```python
from build123d import *

# Parameters (mm, degrees)
SKETCH1_W           = 3
SKETCH1_H           = 30
BOSS_EXTRUDE1_DEPTH = 3


with BuildPart() as part:
    # Sketch1 → Boss-Extrude1 (new body)
    with BuildSketch(Plane.XY):
        Polygon((-90, 0), (-86.5, 0), (-86.5, 3), (-70, 3), (-70, 35), (-8, 35), (-8, 3), (-6.5, 3), (-6.5, 0), (17, 0), (17, 3), (0, 59), (-3, 59), (-90, 33), align=None)
        with Locations((-1.5, 31)):
            Rectangle(SKETCH1_W, SKETCH1_H, mode=Mode.SUBTRACT)
    extrude(amount=BOSS_EXTRUDE1_DEPTH)


solid = part.part
```
Work out the finished part from the listing and answer in its coordinate system (mm). A direction names the side the tool comes from. Coordinates: 2 decimals unless noted, no trailing zeros. Loops run counter-clockwise (first coordinate to the right, second up) from the corner with the lowest first, then second, coordinate; pieces in that order, holes last. Notation, with made-up numbers: (57, 25.25) - (101, 25.25) arc R26 cw to (101, 57.25) - close; hole circle Ø6 at (73.5, -30). An arc over 180 degrees is marked (long way). Use a Markdown table: item, result.
Item 1: For faces 4 (the flat face through (-78, 3, 1)), 5 (the flat face through (-3, 31, 1)), 6 (the flat face through (-88, 0, 1)), determine the directions among +Z, -Z, +X, -X, +Y, -Y from which every point of the face is accessible in a straight line to the end or side of a thin tool.
Evaluation:
| item | result |
|---|---|
| face 4 | +Z, -Z, -Y |
| face 5 | +Z, -Z |
| face 6 | +Z, -Z, +X, -X, -Y |
Item 2: Find section D-D, the plane y = 5.5. Determine the outline of the cut face in (x, z), and give its area (3 significant figures).
Evaluation:
| item | result |
|---|---|
| outline | (-90, 0) - (-70, 0) - (-70, 3) - (-90, 3) - close; (-8, 0) - (16.24, 0) - (16.24, 3) - (-8, 3) - close |
| area | 133 mm2 |
Item 3: The mould has two halves that part along X. Classify faces 1 (the flat face through (-1, 59, 1)), 2 (the flat face through (-86.5, 1, 1)), 3 (the flat face through (17, 1, 1)): +X half, -X half, draft (parallel to the pull), parting line (faces both ways), or undercut.
Evaluation:
| item | result |
|---|---|
| face 1 | draft |
| face 2 | undercut |
| face 3 | +X half |
Item 4: Find section B-B, the plane y = 25. Determine the outline of the cut face in (x, z), and give its area (3 significant figures).
Evaluation:
| item | result |
|---|---|
| outline | (-90, 0) - (-70, 0) - (-70, 3) - (-90, 3) - close; (-8, 0) - (-3, 0) - (-3, 3) - (-8, 3) - close; (0, 0) - (10.32, 0) - (10.32, 3) - (0, 3) - close |
| area | 106 mm2 |
Item 5: Consider probe 1 along X at (y, z) = (28, 1.5); probe 2 along X at (y, z) = (27, 0.7); probe 3 along Y at (x, z) = (-82.5, 2.65). Determine where each line is inside the solid, lowest interval first. Write a range as from..to.
Evaluation:
| item | result |
|---|---|
| probe 1 | x = -90..-70, -8..-3, 0..9.41 |
| probe 2 | x = -90..-70, -8..-3, 0..9.71 |
| probe 3 | y = 3..35.24 |
Item 6: Given pin 1 Ø1.2 at (x, z) = (-7.5, 1) entering from -Y; pin 2 Ø0.9 at (y, z) = (27, 1) entering from +X; pin 3 Ø1.5 at (x, z) = (-68.5, 1.5) entering from -Y, each flat-ended and moving along its own axis, determine where each tip first touches the part or whether it passes through.
Evaluation:
| item | result |
|---|---|
| pin 1 | stops at y = 3 |
| pin 2 | stops at x = 9.85 |
| pin 3 | stops at y = 35 |
Item 7: Find section C-C, the plane y = 13. Determine the outline of the cut face in (x, z).
Evaluation:
| item | result |
|---|---|
| outline | (-90, 0) - (-70, 0) - (-70, 3) - (-90, 3) - close; (-8, 0) - (13.96, 0) - (13.96, 3) - (-8, 3) - close |
Item 8: Find section A-A, the plane z = 2.4. Determine the outline of the cut face in (x, y).
Evaluation:
| item | result |
|---|---|
| outline | (-90, 0) - (-86.5, 0) - (-86.5, 3) - (-70, 3) - (-70, 35) - (-8, 35) - (-8, 3) - (-6.5, 3) - (-6.5, 0) - (17, 0) - (17, 3) - (0, 59) - (-3, 59) - (-90, 33) - close; hole (-3, 16) - (0, 16) - (0, 46) - (-3, 46) - close |
